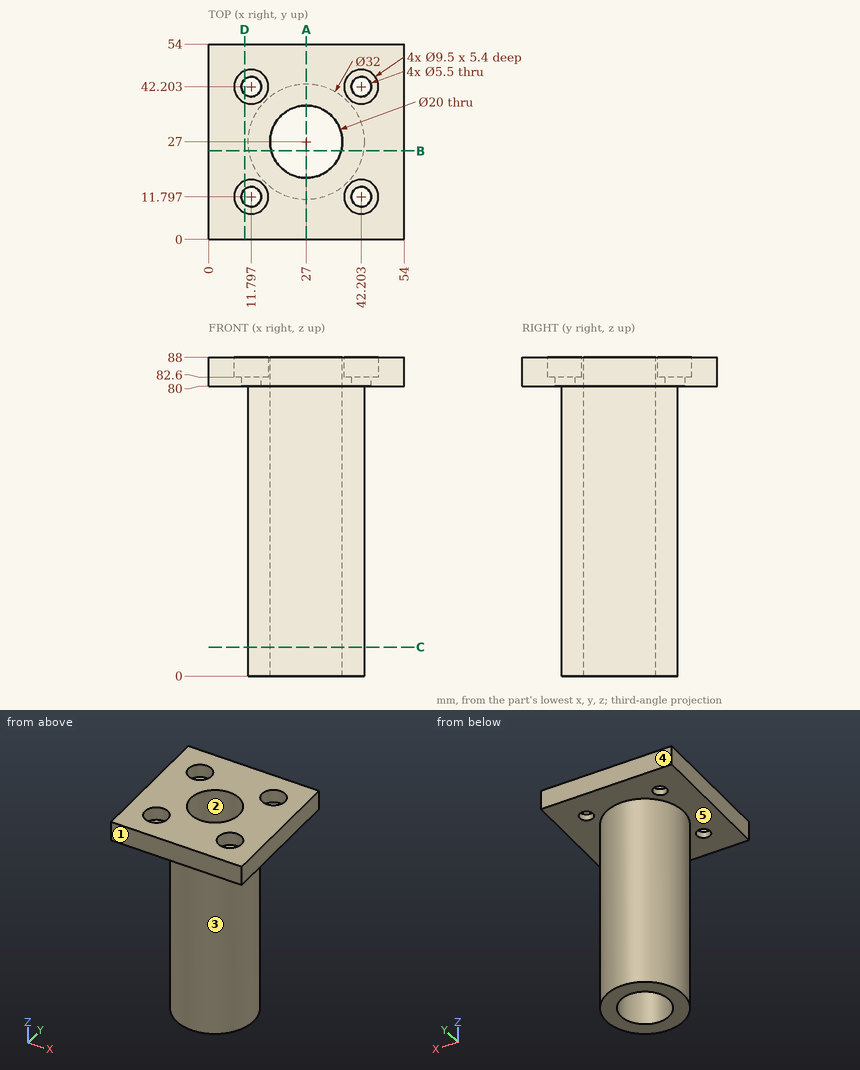
Can you work these out from the drawing? Everything is in mm from the part's minimum corner. A direction names the side the tool comes from. Round coordinates to 2 decimals unless told otherwise and drop trailing zeros. Write each loop counter-clockwise with the first axis right and the second up, starting at its lowest first coordinate (ties: lowest second). Pieces come first, ordered by that corner, then holes.
1. Suppose I cut it at B-B (y = 24.5). List the corners of the cut face in (x, z) for me, and give its area (3 significant figures).
2. For the marked faces 4 and 5, which set-ups out of +Z, -Z, +X, -X, +Y, -Y let a thin tool reach every point of the face, with its end or its side?
3. Suppose I cut it at C-C (z = 8). List the corners of the cut face in (x, y) for me.
4. If we mould it in two halves opening along X, with no side actions, what happens to the marked faces 1, 2 and 3? For each: released by +X, released by -X, zero draft, split by the parting line, or undercut.
5. Suppose I cut it at D-D (x = 10). List the corners of the cut face in (y, z) for me.
6. Will these pins go through, and if not, where does the flat tip stop? pin 1 Ø3 at (y, z) = (45.5, 40.5) entering from +X; pin 2 Ø10.5 at (x, y) = (42, 14) entering from +Z; pin 3 Ø4 at (x, y) = (48, 28) entering from -Z; pin 4 Ø10 at (y, z) = (44, 11) entering from -X.
7. I need wall thicknesses on L1, parallel to Y at x = 9.5, z = 83 (1 decimal); L2, parallel to Y at x = 27, z = 62. Which ranges of each line are inside material? Lowest first, please.
8. Suppose I cut it at A-A (x = 27). List the corners of the cut face in (y, z) for me, and give its area (3 significant figures).
Answer sheet:
1. outline: (0, 80) - (11.2, 80) - (11.2, 0) - (17.32, 0) - (17.32, 88) - (0, 88) - close; (36.68, 0) - (42.8, 0) - (42.8, 80) - (54, 80) - (54, 88) - (36.68, 88) - close
1. area: 1,260 mm2
2. face 4: +Z, -Z, +X, -X, +Y
2. face 5: -Z
3. outline: circle Ø32 at (27, 27); hole circle Ø20 at (27, 27)
4. face 1: zero draft
4. face 2: undercut
4. face 3: split by the parting line
5. outline: (0, 80) - (9.72, 80) - (9.72, 82.6) - (7.4, 82.6) - (7.4, 88) - (0, 88) - close; (13.88, 80) - (40.12, 80) - (40.12, 82.6) - (37.81, 82.6) - (37.81, 88) - (16.19, 88) - (16.19, 82.6) - (13.88, 82.6) - close; (44.28, 80) - (54, 80) - (54, 88) - (46.6, 88) - (46.6, 82.6) - (44.28, 82.6) - close
6. pin 1: passes through
6. pin 2: stops at z = 88
6. pin 3: stops at z = 80
6. pin 4: stops at x = 16.42
7. L1: y = 0 to 7.6, 16 to 38, 46.4 to 54
7. L2: y = 11 to 17, 37 to 43
8. outline: (0, 80) - (11, 80) - (11, 0) - (17, 0) - (17, 88) - (0, 88) - close; (37, 0) - (43, 0) - (43, 80) - (54, 80) - (54, 88) - (37, 88) - close
8. area: 1,230 mm2
